Autodesk Inventor part; units mm, degrees
ref_plane "YZ Plane" through (0, 0, 0) normal (1, 0, 0) x (0, 1, 0)
ref_plane "XZ Plane" through (0, 0, 0) normal (0, 1, 0) x (-1, 0, 0)
ref_plane "XY Plane" through (0, 0, 0) normal (0, 0, 1) x (1, 0, 0)
sketch "Sketch3" plane through (0, 0, 0) normal (0, 1, 0) x (-1, 0, 0)
  circle A0 centre (0, 0) radius 33
  circle A1 centre (0, 0) radius 8
  line L0 (0, 0) -> (32, 0) construction
  line L1 (0, 0) -> (34, 0) construction
  line L2 (24.0416, -24.0416) -> (20.5061, -20.5061)
  line L3 (0, 0) -> (34, 0) construction
  line L4 (0, 0) -> (22.2739, 0)
  line L5 (0, 0) -> (21, 0)
  circle A2 centre (21, 0) radius 8
  circle A3 centre (10.5, 18.1865) radius 8
  circle A4 centre (-10.5, 18.1865) radius 8
  circle A5 centre (-21, 0) radius 8
  circle A6 centre (-10.5, -18.1865) radius 8
  circle A7 centre (10.5, -18.1865) radius 8
  line L6 (0, 0) -> (0, -34)
  dimension "d15" = 66
  dimension "d17" = 16
  dimension "d25" = 34
  dimension "d27" = 5
  dimension "d31" = 21
  dimension "d32" = 16
  dimension "d35" = 360
  dimension "d39" = 34
extrude "Extrusion1" add sketch "Sketch3" along normal blind 2
properties part number "separator"
Can you work these out from the model? Positions are in its coordinate system, mm. Round coordinates to 2 decimals unless told otherwise and drop trailing zeros. Loops run counter-clockwise (first coordinate to the right, second up) from the corner with the lowest first, then second, coordinate; pieces in that order, holes last.
Item 1: Suppose I cut it at D-D, the plane y = 0.6. Write out the boundary of the cut face in (x, z).
Item 2: If we mould it in two halves opening along X, with no side actions, what happens to faces 1 (the cylindrical face through (-30.5, 1, 12.6)), 2 (the flat face through (-7, 2, -7)), 3 (the cylindrical face through (11.54, 0.99, -26.12))? For each: +X half, -X half, draft (parallel to the pull), parting line (faces both ways), or undercut.
Item 3: Suppose I cut it at B-B, the plane x = 6. Write out the boundary of the cut face in (y, z), then the cut area to 3 significant figures.
Item 4: Suppose I cut it at A-A, the plane z = 0. Write out the boundary of the cut face in (x, y).
Item 5: Suppose I cut it at C-C, the plane x = 22. Write out the boundary of the cut face in (y, z), then the cut area to 3 significant figures.
Item 6: Will this pin go through, and if not, where does the flat tip stop? pin 1 Ø1 at (y, z) = (1, 2) entering from +X.
Item 7: Please list where these lines run through material, in increasing order: L1, parallel to X at y = 0.9, z = 6; L2, parallel to X at y = 0.8, z = 11; L3, parallel to Z at x = 10.5, y = 1.45.
Reported:
1. outline: circle Ø66 at (0, 0); hole circle Ø16 at (-21, 0); hole circle Ø16 at (-10.5, -18.19); hole circle Ø16 at (-10.5, 18.19); hole circle Ø16 at (0, 0); hole circle Ø16 at (10.5, -18.19); hole circle Ø16 at (10.5, 18.19); hole circle Ø16 at (21, 0)
2. face 1: parting line
2. face 2: draft
2. face 3: undercut
3. outline: (0, -32.45) - (2, -32.45) - (2, -24.8) - (0, -24.8) - close; (0, -11.57) - (2, -11.57) - (2, -5.29) - (0, -5.29) - close; (0, 5.29) - (2, 5.29) - (2, 11.57) - (0, 11.57) - close; (0, 24.8) - (2, 24.8) - (2, 32.45) - (0, 32.45) - close
3. area: 55.7 mm2
4. outline: (-33, 0) - (-29, 0) - (-29, 2) - (-33, 2) - close; (-13, 0) - (-8, 0) - (-8, 2) - (-13, 2) - close; (8, 0) - (13, 0) - (13, 2) - (8, 2) - close; (29, 0) - (33, 0) - (33, 2) - (29, 2) - close
5. outline: (0, -24.6) - (2, -24.6) - (2, -7.94) - (0, -7.94) - close; (0, 7.94) - (2, 7.94) - (2, 24.6) - (0, 24.6) - close
5. area: 66.6 mm2
6. pin 1: stops at x = 32.97
7. L1: x = -32.45 to -26.29, -15.71 to -5.29, 5.29 to 15.71, 26.29 to 32.45
7. L2: x = -31.11 to -14.01, -6.99 to 6.99, 14.01 to 31.11
7. L3: z = -31.28 to -26.19, -10.19 to 10.19, 26.19 to 31.28
